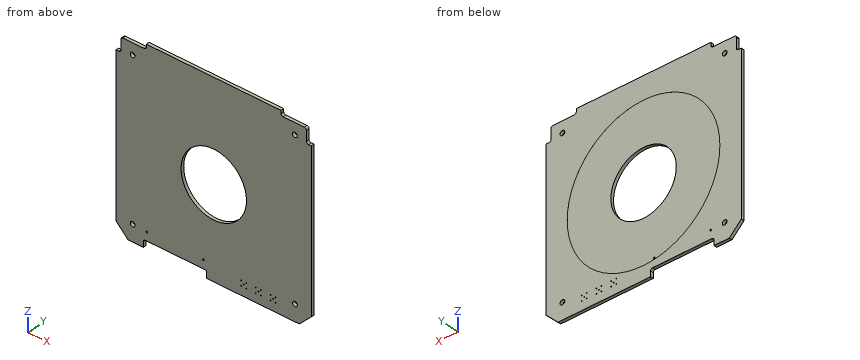
from build123d import *

# Parameters (mm, degrees)
SKETCH1_R                = 0.4
SKETCH1_R_2              = 0.2125
BOSS_EXTRUDE1_DEPTH      = 1.56
M2_CLEARANCE_HOLE2_D     = 2.4
M2_CLEARANCE_HOLE2_DEPTH = 38.1
M2_CLEARANCE_HOLE2_TIP   = 0.721032743
SKETCH2_R                = 38.5
CUT_EXTRUDE1_DEPTH       = 0.01
SKETCH10_R               = 16.5
CUT_EXTRUDE2_DEPTH       = 10


with BuildPart() as part:
    # Sketch1 → Boss-Extrude1 (new body)
    with BuildSketch(Plane(origin=(0, 0, 0), x_dir=(1, 0, 0), z_dir=(0, 1, 0))):
        with BuildLine():
            Line((-49.356685196, 41.604788024), (-43.256685196, 47.704788024))
            Line((-43.256685196, 47.704788024), (-35.556685196, 47.704788024))
            Line((-35.556685196, 47.704788024), (-35.556685196, 45.004788024))
            ThreePointArc((-35.556685196, 45.004788024), (-35.263791977, 44.297681243), (-34.556685196, 44.004788024))
            Line((-34.556685196, 44.004788024), (-4.556685196, 44.004788024))
            ThreePointArc((-4.556685196, 44.004788024), (-3.849578415, 44.297681243), (-3.556685196, 45.004788024))
            Line((-3.556685196, 45.004788024), (-3.556685196, 47.704788024))
            Line((-3.556685196, 47.704788024), (43.143314804, 47.704788024))
            Line((43.143314804, 47.704788024), (49.243314804, 41.604788024))
            Line((49.243314804, 41.604788024), (49.243314804, -37.995211976))
            Line((49.243314804, -37.995211976), (47.743314804, -37.995211976))
            ThreePointArc((47.743314804, -37.995211976), (47.036208023, -38.288105194), (46.743314804, -38.995211976))
            Line((46.743314804, -38.995211976), (46.743314804, -44.095211976))
            ThreePointArc((46.743314804, -44.095211976), (46.450421585, -44.802318757), (45.743314804, -45.095211976))
            Line((45.743314804, -45.095211976), (34.943314804, -45.095211976))
            ThreePointArc((34.943314804, -45.095211976), (34.236208023, -45.388105194), (33.943314804, -46.095211976))
            Line((33.943314804, -46.095211976), (33.943314804, -47.595211976))
            Line((33.943314804, -47.595211976), (-34.056685196, -47.595211976))
            Line((-34.056685196, -47.595211976), (-34.056685196, -46.095211976))
            ThreePointArc((-34.056685196, -46.095211976), (-34.349578415, -45.388105194), (-35.056685196, -45.095211976))
            Line((-35.056685196, -45.095211976), (-45.856685196, -45.095211976))
            ThreePointArc((-45.856685196, -45.095211976), (-46.563791977, -44.802318757), (-46.856685196, -44.095211976))
            Line((-46.856685196, -44.095211976), (-46.856685196, -38.995211976))
            ThreePointArc((-46.856685196, -38.995211976), (-47.149578415, -38.288105194), (-47.856685196, -37.995211976))
            Line((-47.856685196, -37.995211976), (-49.356685196, -37.995211976))
            Line((-49.356685196, -37.995211976), (-49.356685196, 41.604788024))
        make_face()
        with Locations(Location((-33.826685196, 39.744788024, 0), (0, 0, 270))):
            Circle(SKETCH1_R, mode=Mode.SUBTRACT)
        with Locations(Location((-5.276685196, 39.744788024, 0), (0, 0, 270))):
            Circle(SKETCH1_R, mode=Mode.SUBTRACT)
        with Locations(Location((29.883314804, 42.004788024, 0), (0, 0, 270))):
            Circle(SKETCH1_R_2, mode=Mode.SUBTRACT)
        with Locations(Location((28.613314804, 43.274788024, 0), (0, 0, 270))):
            Circle(SKETCH1_R_2, mode=Mode.SUBTRACT)
        with Locations(Location((31.153314804, 43.274788024, 0), (0, 0, 270))):
            Circle(SKETCH1_R_2, mode=Mode.SUBTRACT)
        with Locations(Location((31.153314804, 40.734788024, 0), (0, 0, 270))):
            Circle(SKETCH1_R_2, mode=Mode.SUBTRACT)
        with Locations(Location((28.613314804, 40.734788024, 0), (0, 0, 270))):
            Circle(SKETCH1_R_2, mode=Mode.SUBTRACT)
        with Locations(Location((22.483314804, 42.004788024, 0), (0, 0, 270))):
            Circle(SKETCH1_R_2, mode=Mode.SUBTRACT)
        with Locations(Location((21.213314804, 43.274788024, 0), (0, 0, 270))):
            Circle(SKETCH1_R_2, mode=Mode.SUBTRACT)
        with Locations(Location((23.753314804, 43.274788024, 0), (0, 0, 270))):
            Circle(SKETCH1_R_2, mode=Mode.SUBTRACT)
        with Locations(Location((23.753314804, 40.734788024, 0), (0, 0, 270))):
            Circle(SKETCH1_R_2, mode=Mode.SUBTRACT)
        with Locations(Location((21.213314804, 40.734788024, 0), (0, 0, 270))):
            Circle(SKETCH1_R_2, mode=Mode.SUBTRACT)
        with Locations(Location((15.083314804, 42.004788024, 0), (0, 0, 270))):
            Circle(SKETCH1_R_2, mode=Mode.SUBTRACT)
        with Locations(Location((13.813314804, 43.274788024, 0), (0, 0, 270))):
            Circle(SKETCH1_R_2, mode=Mode.SUBTRACT)
        with Locations(Location((16.353314804, 43.274788024, 0), (0, 0, 270))):
            Circle(SKETCH1_R_2, mode=Mode.SUBTRACT)
        with Locations(Location((16.353314804, 40.734788024, 0), (0, 0, 270))):
            Circle(SKETCH1_R_2, mode=Mode.SUBTRACT)
        with Locations(Location((13.813314804, 40.734788024, 0), (0, 0, 270))):
            Circle(SKETCH1_R_2, mode=Mode.SUBTRACT)
    extrude(amount=BOSS_EXTRUDE1_DEPTH)

    # M2 Clearance Hole2
    with Locations(Plane(origin=(0, 1.56, 0), x_dir=(1, 0, 0), z_dir=(0, 1, 0))):
        with Locations((-40.929491149, 39.39737116), (40.929491149, 39.39737116), (40.929491149, -39.39737116), (-40.929491149, -39.39737116)):
            Hole(M2_CLEARANCE_HOLE2_D / 2, depth=M2_CLEARANCE_HOLE2_DEPTH)
            with Locations((0, 0, -(M2_CLEARANCE_HOLE2_DEPTH + M2_CLEARANCE_HOLE2_TIP / 2))):  # 118° drill point
                Cone(0, M2_CLEARANCE_HOLE2_D / 2, M2_CLEARANCE_HOLE2_TIP, mode=Mode.SUBTRACT)

    # Sketch2 → Cut-Extrude1 (cut)
    with BuildSketch(Plane(origin=(0, 1.56, 0), x_dir=(1, 0, 0), z_dir=(0, 1, 0))):
        with Locations(Location((0, 2.34737116, 0), (0, 0, 270))):
            Circle(SKETCH2_R)
    extrude(amount=-CUT_EXTRUDE1_DEPTH, mode=Mode.SUBTRACT)

    # Sketch10 → Cut-Extrude2 (cut)
    with BuildSketch(Plane(origin=(0, 1.55, 0), x_dir=(1, 0, 0), z_dir=(0, 1, 0))):
        with Locations(Location((0, 2.34737116, 0), (0, 0, 270))):
            Circle(SKETCH10_R)
    extrude(amount=-CUT_EXTRUDE2_DEPTH, mode=Mode.SUBTRACT)


solid = part.part
Can you work these out from the model? Positions are in its coordinate system, mm. Round coordinates to 2 decimals unless told otherwise and drop trailing zeros. Write each question's results on one line, items separated by ' | '. Start each with the question number.
1) Please list where these lines run through material, in increasing order: line 1 (Z direction, x = -41, y = 1.45); line 2 (Y direction, x = -11.5, z = -22); line 3 (Z direction, x = 40, y = 0.6).
2) For pin 1 Ø3 at (x, z) = (-36, 2) entering from +Y; pin 2 Ø0.8 at (y, z) = (1, -46) entering from +X; pin 3 Ø0.8 at (y, z) = (0.5, -47) entering from -X, each with a flat end and sliding along its axis, tell me the tip position at first contact or that it passes through.
3) Suppose I cut it at D-D (y = 1.25). Give the number of separate pieces and of enclosed holes in the cut face, and give its area (3 significant figures).
Here are the results:
1) line 1: z = -47.7 to -40.6, -38.2 to 38.2, 40.6 to 45.1 | line 2: y = 0 to 1.55 | line 3: z = -47.7 to -40.16, -38.64 to 38.64, 40.16 to 45.1
2) pin 1: stops at y = 1.55 | pin 2: stops at x = 45.25 | pin 3: stops at x = -44.36
3) separate pieces: 1 | enclosed holes: 22 | area: 8,250 mm2
